from build123d import *

# Parameters (mm, degrees)
ESQUISSE2_R                  = 1
ENL_V_MAT_EXTRU_1_DEPTH      = 15
ENL_V_MAT_EXTRU_1_DEPTH_BACK = 15


with BuildPart() as part:
    # Esquisse1 → Révolution1 (revolve)
    with BuildSketch(Plane.XY, mode=Mode.PRIVATE) as r_volution1_sk:
        Polygon((0, 0), (0, 7.65), (1, 8.65), (165, 8.65), (165, 13), (166, 14), (191, 14), (192, 13), (192, 0), align=None)
    revolve(r_volution1_sk.sketch.rotate(Axis((0, 0, 0), (1, 0, 0)), 180), axis=Axis((0, 0, 0), (1, 0, 0)))  # turned: the seam where the file's is

    # Esquisse2 → Enlèv. mat.-Extru.1 (cut, two sides)
    with BuildSketch(Plane.XY) as enl_v_mat_extru_1_sk:
        with Locations((4, 0)):
            Circle(ESQUISSE2_R)
    extrude(amount=ENL_V_MAT_EXTRU_1_DEPTH, mode=Mode.SUBTRACT)
    extrude(enl_v_mat_extru_1_sk.sketch, amount=-ENL_V_MAT_EXTRU_1_DEPTH_BACK, mode=Mode.SUBTRACT)


solid = part.part
Geometry check sheet. Reference: the model listing, model coordinates, mm. A direction names the side the tool comes from. Round coordinates to 2 decimals unless told otherwise and drop trailing zeros. Write each loop counter-clockwise with the first axis right and the second up, starting at its lowest first coordinate (ties: lowest second). Pieces come first, ordered by that corner, then holes.
Item 1: Material ranges on line 1 along X through (y, z) = (0, 5); line 2 along X through (y, z) = (5.5, -8); line 3 along Y through (x, z) = (4, -0.5), recorded low to high.
Determined:
line 1: x = 0 to 3, 5 to 192
line 2: x = 165 to 192
line 3: y = -8.64 to -1, 1 to 8.64
Item 2: Section check B-B (x = 36.5). Record the boundary of the cut face in (y, z), plus the area to 3 significant figures.
Determined:
outline: circle Ø17.3 at (0, 0)
area: 235 mm2
Item 3: Access from +Z, -Z, +X, -X, +Y, -Y to the whole of each face (thin tool, end or side, straight path). Record for faces 1 (the face through (84.15, -8.25, -2.6)), 2 (the face through (178.675, -12.932, 5.362)).
Determined:
face 1: -X
face 2: +X, -X
Item 4: Section check A-A (z = 0). Record the boundary of the cut face in (x, y), plus the area to 3 significant figures.
Determined:
outline: (0, -7.65) - (1, -8.65) - (165, -8.65) - (165, -13) - (166, -14) - (191, -14) - (192, -13) - (192, 13) - (191, 14) - (166, 14) - (165, 13) - (165, 8.65) - (1, 8.65) - (0, 7.65) - close; hole circle Ø2 at (4, 0)
area: 3,600 mm2
Item 5: Go/stop test with flat-tipped pins: pin 1 Ø4 at (x, z) = (121, -7) entering from +Y; pin 2 Ø10 at (x, y) = (55, -7.5) entering from +Z; pin 3 Ø6 at (x, y) = (104, 3) entering from +Z; pin 4 Ø1.8 at (x, y) = (4, 0) entering from -Z. Record where each tip stops, or that it passes through.
Determined:
pin 1: stops at y = 7.06
pin 2: stops at z = 8.28
pin 3: stops at z = 8.65
pin 4: passes through
